Read the model definition and answer for the solid it produces. Units are mm, in the model's axes. Face numbers are marked on the shaded views. A direction names the side the tool comes from. Coordinates: 2 decimals unless noted, no trailing zeros. Loops run counter-clockwise (first coordinate to the right, second up) from the corner with the lowest first, then second, coordinate; pieces in that order, holes last. Notation, with made-up numbers: M 80,-38 L 107,-38 A31 cw 107,-1 Z; hole C 51,61 d4. An arc over 180 degrees is marked long. Use one line per item in the form item = value. Start each with the question number.
1. The part is cut by section D-D (y = 9.5). Give the vertices of the cut face in (x, z).
2. The part is cut by section C-C (x = 12.5). Give the vertices of the cut face in (y, z).
3. For a pull along Z with two mould halves and no side action, classify the marked faces 1, 2, 3 and 4 as released by +Z, released by -Z, zero draft, split by the parting line, or undercut.
4. The part is cut by section A-A (x = 7). Give the vertices of the cut face in (y, z), plus the area to 3 significant figures.
5. Flat-ended cylindrical pins translate along their axes: pin 1 (2 mm diameter, centred on x = 7, y = -2.5, fed in from -Z); pin 2 (4.5 mm diameter, centred on x = 6, y = 2, fed in from -Z); pin 3 (1.6 mm diameter, centred on x = 7.5, y = 1.5, fed in from +Z). Find the tip coordinate at first contact, or state that the pin passes through.
6. Find the intervals of material crossed by probe 1 along X at (y, z) = (20, 27.5); probe 2 along Z at (x, y) = (7, 18.75); probe 3 along Z at (x, y) = (10, 0), in increasing order. Write a range as [from, to].
7. A tool of negligible diameter and unlimited length cuts with its end or side. For the marked faces 5, 6 and 7, from which of +Z, -Z, +X, -X, +Y, -Y can it reach the whole face along a straight path? Write none if from no direction.
8. The part is cut by section B-B (z = 0). Give the vertices of the cut face in (x, y).
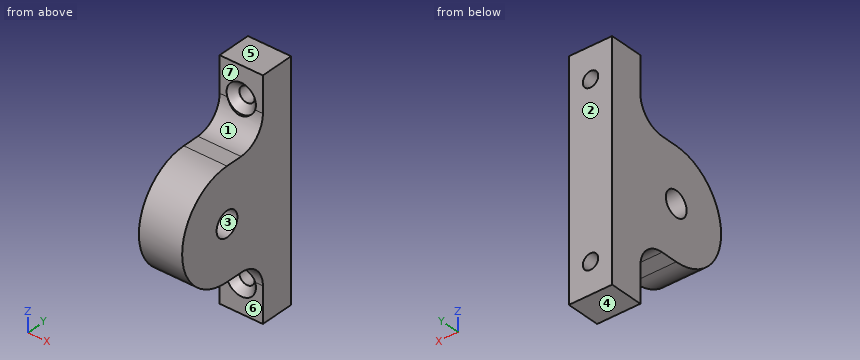
Autodesk Inventor part; units mm, degrees
ref_plane "YZ Plane" through (0, 0, 0) normal (1, 0, 0) x (0, 1, 0)
ref_plane "XZ Plane" through (0, 0, 0) normal (0, 1, 0) x (-1, 0, 0)
ref_plane "XY Plane" through (0, 0, 0) normal (0, 0, 1) x (1, 0, 0)
sketch "Sketch1" plane through (0, 0, 0) normal (1, 0, 0) x (0, 1, 0)
  circle A0 centre (0, 0) radius 4.05
  circle A1 centre (0, 0) radius 17.5
  line L0 (0, 17.5) -> (25, 17.5)
  line L1 (0, -17.5) -> (25, -17.5)
  line L2 (25, -17.5) -> (25, 17.5)
  dimension "d0" = 8.1
  dimension "d1" = 35
  dimension "d2" = 25
  dimension "d3" = 25
extrude "Extrusion1" add sketch "Sketch1" along normal blind 14
ref_plane "Work Plane1" through (0, 0, 0) normal (0, 0, -1) x (-1, 0, 0)
sketch "Sketch2" plane through (14, 0, 0) normal (1, 0, 0) x (0, 0, -1)
  line L0 (17.5, 25) -> (-17.5, 25)
  line L1 (17.5, 25) -> (37.5, 25)
  line L2 (37.5, 25) -> (37.5, 14)
  line L3 (37.5, 14) -> (17.5, 14)
  line L4 (17.5, 14) -> (17.5, 25)
  point P0 (0, 0)
  dimension "d6" = 20
  dimension "d7" = 11
extrude "Extrusion2" add sketch "Sketch2" against normal blind 14
fillet "Fillet1" radius 8.5 1 edges at (7, 14, -17.5)
sketch "Sketch3" plane through (0, 14, -37.5) normal (0, -1, 0) x (1, 0, 0)
  line L0 (14, 0) -> (0, 0) construction
  line L1 (7, 0) -> (7, 10) construction
  point P0 (0, 37.5)
  dimension "d11" = 10
hole "Hole1" at (7, 14, -27.5) direction (0, 1, 0) diameter 5 end through all countersink diameter 9.5 countersink angle 90
sketch "Sketch4" plane through (0, 14, -37.5) normal (0, -1, 0) x (1, 0, 0)
  arc A0 (2.4931, 11.5) -> (11.5069, 11.5) centre (7, 10) ccw
  circle A1 centre (7, 10) radius 4.75
  point P0 (0, 37.5)
  point P1 (11.5069, 11.5)
extrude "Extrusion3" cut sketch "Sketch4" along normal blind 14
mirror "Mirror1" about plane through (0, 0, 0) normal (0, 0, -1) of "Hole1", "Extrusion3", "Extrusion2", "Fillet1"
properties part number "Passive Wheel 8mm bore bracket"
Computed values:
q1.outline = M 0,-18.5 L 14,-18.5 L 14,18.5 L 0,18.5 Z
q2.outline = M 0,-17.5 L 5.5,-17.5 A8.5 cw 14,-26 L 14,-37.5 L 25,-37.5 L 25,37.5 L 14,37.5 L 14,26 A8.5 cw 5.5,17.5 L 0,17.5 A17.5 ccw Z; hole C 0,0 d8.1
q3.face_1 = released by +Z
q3.face_2 = zero draft
q3.face_3 = undercut
q3.face_4 = released by -Z
q4.outline = M 0,-17.5 L 5.5,-17.5 A8.5 cw 13.35,-22.75 L 14,-22.75 L 16.25,-25 L 25,-25 L 25,25 L 16.25,25 L 14,22.75 L 13.35,22.75 A8.5 cw 5.5,17.5 L 0,17.5 A17.5 ccw Z; M 14,-37.5 L 25,-37.5 L 25,-30 L 16.25,-30 L 14,-32.25 Z; M 14,32.25 L 16.25,30 L 25,30 L 25,37.5 L 14,37.5 Z; hole C 0,0 d8.1
q4.area = 1,650 mm²
q5.pin_1 = -17.44
q5.pin_2 = -17.5
q5.pin_3 = 17.5
q6.probe_1 = [0, 4.5], [9.5, 14]
q6.probe_2 = [-37.5, -30], [-25, 25], [30, 37.5]
q6.probe_3 = [-17.5, -4.05], [4.05, 17.5]
q7.face_5 = +Z, +X, -X, +Y, -Y
q7.face_6 = -Z, +X, -X, -Y
q7.face_7 = +Z, +X, -X, -Y
q8.outline = M 0,-17.5 L 14,-17.5 L 14,-4.05 L 0,-4.05 Z; M 0,4.05 L 14,4.05 L 14,25 L 0,25 Z
